Check sheet for the modelled part. Datum: model origin and axes. Units: mm. Face numbers are marked on the shaded views. Give positions to 0.01 mm unless a question says otherwise; leave off trailing zeros. Answer in a Markdown table with one row per item.
Autodesk Inventor part; units mm, degrees
ref_plane "YZ Plane" through (0, 0, 0) normal (1, 0, 0) x (0, 1, 0)
ref_plane "XZ Plane" through (0, 0, 0) normal (0, 1, 0) x (-1, 0, 0)
ref_plane "XY Plane" through (0, 0, 0) normal (0, 0, 1) x (1, 0, 0)
sketch "Sketch1" plane through (0, 0, 0) normal (0, 0, 1) x (1, 0, 0)
  circle A0 centre (0, 0) radius 5.5563
  circle A1 centre (0, 0) radius 9.525
  dimension "d0" = 11.1125
extrude "Extrusion1" add sketch "Sketch1" along normal blind 1.5875
chamfer "Chamfer1" distance 0.127 distance2 1.5875 1 edges at (-9.525, 0, 1.5875) measured on face at (9.4941, -0.7664, 1.0583)
chamfer "Chamfer2" distance 1.5875 distance2 0.127 1 edges at (-9.525, 0, 0) measured on face at (8.1098, -0.7598, 0)
chamfer "Chamfer3" distance 0.127 angle 45 2 edges at (-5.5563, 0, 0) (-5.5563, 0, 1.5875)
properties part number "trim washer" material "Stainless Steel"
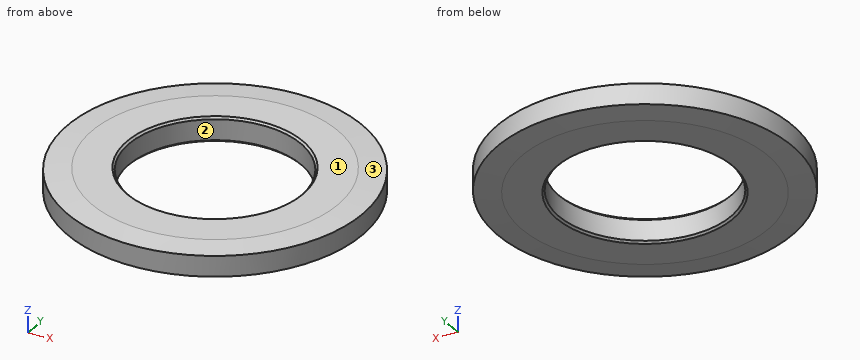
(1) Gauge pin test, flat end, axial feed: P1, Ø10, axis at x = 0, y = 0, coming from the -Z side. Record the tip position at first contact, or that the pin passes through.
Geometry says:
| item | result |
|---|---|
| P1 | through |
(2) Mould release check, pull along Y, two halves, no side actions. Record for the marked faces 1, 2 and 3: pulls with the +Y half, pulls with the -Y half, needs draft (parallel to the pull), parting line crosses it, or undercut.
Geometry says:
| item | result |
|---|---|
| face 1 | needs draft |
| face 2 | undercut |
| face 3 | parting line crosses it |
(3) Thickness scan on L1, parallel to Y at x = 0, z = 0.75 (3 decimals); L2, parallel to X at y = -0.25, z = 0.4; L3, parallel to Y at x = -1.5, z = 1.1. Record the ranges inside material, lowest first.
Geometry says:
| item | result |
|---|---|
| L1 | -9.525 to -5.556, 5.556 to 9.525 |
| L2 | -9.52 to -5.55, 5.55 to 9.52 |
| L3 | -9.41 to -5.35, 5.35 to 9.41 |
